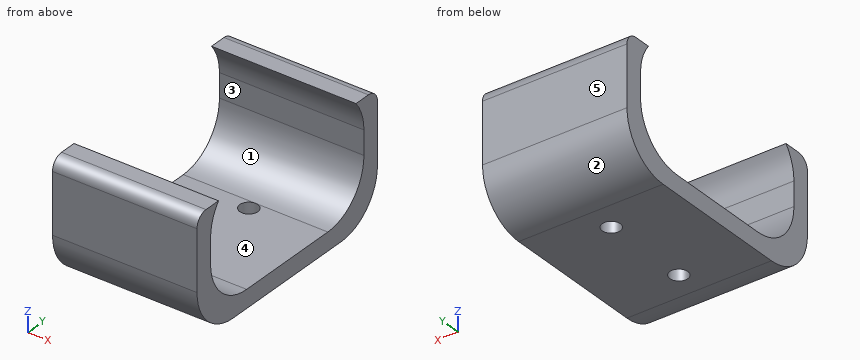
from build123d import *

# Parameters (mm, degrees)
F1_DEPTH = 24
F2_R     = 1.5
F3_DEPTH = 5


with BuildPart() as f1:
    # F0 (on Right) → F1 (new body)
    with BuildSketch(Plane.YZ):
        with BuildLine():
            ThreePointArc((0, 8), (2.343146, 2.343146), (8, 0))
            Line((8, 0), (32, 0))
            ThreePointArc((32, 0), (37.656854, 2.343146), (40, 8))
            Line((40, 8), (40, 18))
            ThreePointArc((40, 18), (39.414214, 19.414214), (38, 20))
            Line((38, 20), (35.244998, 20))
            ThreePointArc((35.244998, 20), (36.548509, 17.64953), (37, 15))
            Line((37, 15), (37, 11))
            ThreePointArc((37, 11), (34.656854, 5.343146), (29, 3))
            Line((29, 3), (11, 3))
            ThreePointArc((11, 3), (5.343146, 5.343146), (3, 11))
            Line((3, 11), (3, 15))
            ThreePointArc((3, 15), (3.451491, 17.64953), (4.755002, 20))
            Line((4.755002, 20), (2, 20))
            ThreePointArc((2, 20), (0.585786, 19.414214), (0, 18))
            Line((0, 18), (0, 8))
        make_face()
    extrude(amount=F1_DEPTH)

    # F2 (on Top) → F3 (cut)
    with BuildSketch(Plane.XY):
        with Locations((12, 12.5)):
            Circle(F2_R)
        with Locations((12, 27.5)):
            Circle(F2_R)
    extrude(amount=F3_DEPTH, mode=Mode.SUBTRACT)


solid = f1.part
Can you work these out from the model? Positions are in its coordinate system, mm. Face numbers are marked on the shaded views. A direction names the side the tool comes from. Round coordinates to 2 decimals unless told otherwise and drop trailing zeros. Loops run counter-clockwise (first coordinate to the right, second up) from the corner with the lowest first, then second, coordinate; pieces in that order, holes last. Notation, with made-up numbers: (12, 89.5) - (28, 89.5) arc R14 ccw to (28, 105.5) - close; hole circle Ø10 at (35.25, 66). An arc over 180 degrees is marked (long way). Use CSV: the item, a comma, the result in double quotes. Start each with the question number.
1) If we section it at C-C on x = 12.75: Write out the boundary of the cut face in (y, z) (3 decimals).
2) If we section it at D-D on x = 3.5: Write out the boundary of the cut face in (y, z) (3 decimals).
3) We'd pull the mould along Z, two halves only. Please class the marked faces 3, 4 and 5: released by +Z, released by -Z, zero draft, split by the parting line, or undercut.
4) For the marked faces 1 and 2, which set-ups out of +Z, -Z, +X, -X, +Y, -Y let a thin tool reach every point of the face, with its end or its side?
5) Please list where these lines run through material, in increasing order: probe 1 along Y at (x, z) = (17.25, 10.75); probe 2 along X at (y, z) = (12.5, 0.7); probe 3 along Y at (x, z) = (12, 1.55). Write a range as [from, to].
6) If we section it at B-B on y = 12.5: Write out the boundary of the cut face in (x, z).
7) For pin 1 Ø1.5 at (x, y) = (9, 34) entering from -Z, with a flat end and sliding along its axis, tell me the tip position at first contact or that it passes through.
8) If we section it at A-A on z = 11.5: Write out the boundary of the cut face in (x, y).
Geometry results:
1,outline,"(0, 8) arc R8 ccw to (8, 0) - (11.201, 0) - (11.201, 3) - (11, 3) arc R8 cw to (3, 11) - (3, 15) arc R8 cw to (4.755, 20) - (2, 20) arc R2 ccw to (0, 18) - close; (13.799, 0) - (26.201, 0) - (26.201, 3) - (13.799, 3) - close; (28.799, 0) - (32, 0) arc R8 ccw to (40, 8) - (40, 18) arc R2 ccw to (38, 20) - (35.245, 20) arc R8 cw to (37, 15) - (37, 11) arc R8 cw to (29, 3) - (28.799, 3) - close"
2,outline,"(0, 8) arc R8 ccw to (8, 0) - (32, 0) arc R8 ccw to (40, 8) - (40, 18) arc R2 ccw to (38, 20) - (35.245, 20) arc R8 cw to (37, 15) - (37, 11) arc R8 cw to (29, 3) - (11, 3) arc R8 cw to (3, 11) - (3, 15) arc R8 cw to (4.755, 20) - (2, 20) arc R2 ccw to (0, 18) - close"
3,face 3,"undercut"
3,face 4,"released by +Z"
3,face 5,"zero draft"
4,face 1,"+X, -X"
4,face 2,"-Z, +X, -X, +Y"
5,probe 1,"y = [0, 3], [37, 40]"
5,probe 2,"x = [0, 10.5], [13.5, 24]"
5,probe 3,"y = [3.27, 11], [14, 26], [29, 36.73]"
6,outline,"(0, 0) - (10.5, 0) - (10.5, 3) - (0, 3) - close; (13.5, 0) - (24, 0) - (24, 3) - (13.5, 3) - close"
7,pin 1,"stops at z = 0.1"
8,outline,"(0, 0) - (24, 0) - (24, 3) - (0, 3) - close; (0, 37) - (24, 37) - (24, 40) - (0, 40) - close"
